Could you check a few things on this model? Use its own coordinates, in mm. A direction names the side the tool comes from. Give positions to 0.01 mm unless a question says otherwise; leave off trailing zeros. Loops run counter-clockwise (first coordinate to the right, second up) from the corner with the lowest first, then second, coordinate; pieces in that order, holes last. Notation, with made-up numbers: (11.25, 34.5) - (66.25, 34.5) arc R16 cw to (66.25, 59.5) - close; hole circle Ø1 at (26.5, 2.5). An arc over 180 degrees is marked (long way). Use CSV: the item, a comma, the result in double quotes.
Autodesk Inventor part; units mm, degrees
ref_plane "Arbeitsebene1" through (0, 18, 0) normal (0, 1, 0) x (-1, 0, 0)
ref_plane "YZ Plane" through (0, 0, 0) normal (1, 0, 0) x (0, 1, 0)
ref_plane "XY Plane" through (0, 0, 0) normal (0, 0, 1) x (1, 0, 0)
sketch "Skizze1" plane through (0, 0, 0) normal (0, 1, 0) x (-1, 0, 0)
  line L0 (0, 0) -> (14, 0)
  line L1 (14, 0) -> (14, -23)
  line L2 (14, -23) -> (14, -23)
  line L3 (14, -23) -> (14, -33)
  line L4 (14, -33) -> (14, -33)
  line L5 (14, -33) -> (14, -106)
  line L6 (14, -106) -> (18, -106)
  line L7 (18, -106) -> (18, -165)
  line L8 (18, -165) -> (18, -165)
  line L9 (18, -165) -> (18, -171)
  line L10 (18, -171) -> (18, -171)
  line L11 (18, -171) -> (18, -176)
  line L12 (18, -176) -> (0, -176)
  line L13 (0, -176) -> (0, 0)
  point P0 (18, -168)
  point P1 (18, -173.5)
  point P2 (14, -28)
  dimension "d3" = 36
  dimension "d6" = 78
  dimension "d8" = 28
  dimension "d12" = 176
  dimension "d13" = 36
  dimension "d14" = 70
revolve "Umdrehung1" add sketch "Skizze1" angle 360 about axis through (0, 0, -176) along (0, 0, 1)
ref_plane "Arbeitsebene1" through (0, 18, 0) normal (0, 1, 0) x (-1, 0, 0)
sketch "Skizze2" plane through (0, 18, 0) normal (0, 1, 0) x (-1, 0, 0)
  line L0 (18, -106) -> (-18, -106)
  line L1 (18, -176) -> (-18, -176)
  line L2 (14, 0) -> (-14, 0)
  point P0 (0, 0)
  point P1 (0, -168)
  point P2 (0, -176)
  point P3 (0, -14)
  dimension "d16" = 8
  dimension "d17" = 14
hole "Bohrung1" at (0, 18, -168) direction (0, -1, 0) diameter 6 end through all
hole "Bohrung2" at (0, 18, -14) direction (0, -1, 0) diameter 10 end through all
properties part number "18"
1) Which directions (+Z, -Z, +X, -X, +Y, -Y) give clear straight access to the entire face, cutting with the end or side of a thin tool? Please do faces 5 (the cylindrical face through (2.343, 17.847, -141.49)), 6 (the flat face through (-9, 11, -106)).
Answer below:
face 5,"+Z, -Z"
face 6,"+Z"
2) Suppose I cut it at C-C (z = -37). Please give me the cut outline in (x, y), plus the area to 3 significant figures.
Answer below:
outline,"circle Ø28 at (0, 0)"
area,"616 mm2"
3) Suppose I cut it at A-A (x = 0). Please give me the cut outline in (y, z).
Answer below:
outline,"(-18, -176) - (18, -176) - (18, -171) - (-18, -171) - close; (-18, -165) - (18, -165) - (18, -106) - (14, -106) - (14, -19) - (-14, -19) - (-14, -106) - (-18, -106) - close; (-14, -9) - (14, -9) - (14, 0) - (-14, 0) - close"
4) I need wall thicknesses on line 1 along Z through (x, y) = (0, -6); line 2 along Z through (x, y) = (-2, -12.5); line 3 along X through (y, z) = (1, -14). Which ranges of each line are inside material? Lowest first, please.
Answer below:
line 1,"z = -176 to -171, -165 to -19, -9 to 0"
line 2,"z = -176 to -170.24, -165.76 to -18.58, -9.42 to 0"
line 3,"x = -13.96 to -5, 5 to 13.96"
5) I'm going to push flat-ended pins straight in: P1, Ø13, axis at x = 0, z = -14, coming from the +Y side; P2, Ø10, axis at y = -3, z = -91.5, coming from the -X side; P3, Ø8, axis at x = 0, z = -168, coming from the +Y side; P4, Ø3, axis at y = -6, z = -147.5, coming from the -X side. Where does each tip first touch, or does it pass through?
Answer below:
P1,"stops at y = 14"
P2,"stops at x = -14"
P3,"stops at y = 18"
P4,"stops at x = -17.43"
6) Suppose I cut it at D-D (x = -6.5). Please give me the cut outline in (y, z).
Answer below:
outline,"(-16.79, -176) - (16.79, -176) - (16.79, -106) - (12.4, -106) - (12.4, 0) - (-12.4, 0) - (-12.4, -106) - (-16.79, -106) - close"
7) We'd pull the mould along Z, two halves only. Please class faces 1 (the cylindrical face through (-0.9, -0.25, -165.14)), 2 (the flat face through (0, 0, -176)), 3 (the cylindrical face through (-1.5, -0.2, -9.23)), 4 (the flat face through (0, 0, 0)): +Z half, -Z half, draft (parallel to the pull), parting line (faces both ways), or undercut.
Answer below:
face 1,"undercut"
face 2,"-Z half"
face 3,"undercut"
face 4,"+Z half"
8) Suppose I cut it at B-B (y = 0). Please give me the cut outline in (x, z).
Answer below:
outline,"(-18, -176) - (18, -176) - (18, -106) - (14, -106) - (14, 0) - (-14, 0) - (-14, -106) - (-18, -106) - close; hole circle Ø10 at (0, -14); hole circle Ø6 at (0, -168)"
